Autodesk Inventor part; units mm, degrees
ref_plane "YZ Plane" through (0, 0, 0) normal (1, 0, 0) x (0, 1, 0)
ref_plane "XZ Plane" through (0, 0, 0) normal (0, 1, 0) x (-1, 0, 0)
ref_plane "XY Plane" through (0, 0, 0) normal (0, 0, 1) x (1, 0, 0)
sketch "main" plane through (0, 0, 0) normal (0, 0, 1) x (1, 0, 0)
  circle A0 centre (-11.2144, -104.2473) radius 2.1844
  circle A1 centre (1.4856, -104.2473) radius 2.1844
  circle A2 centre (48.9096, 6.9894) radius 2.1844
  circle A3 centre (-26.5889, 92.8058) radius 2.1844
  arc A4 (1.4856, -110.5973) -> (7.2979, -106.8047) centre (1.4856, -104.2473) ccw
  arc A5 (-17.0266, -101.6899) -> (-11.2144, -110.5973) centre (-11.2144, -104.2473) ccw
  line L0 (54.6905, 10.0319) -> (-22.1306, 97.3516)
  line L1 (55.7352, 3.2802) -> (7.2979, -106.8047)
  line L2 (-31.0925, 97.9248) -> (-34.2947, 95.1076)
  line L3 (-33.7837, 110.5973) -> (6.8178, 64.4472)
  line L4 (-17.0266, -101.6899) -> (6.006, -49.3432)
  line L5 (-34.8679, 86.1457) -> (-10.7088, 58.6849)
  arc A6 (-34.2947, 95.1076) -> (-34.8679, 86.1457) centre (-30.1004, 90.34) ccw
  arc A7 (-22.1306, 97.3516) -> (-31.0925, 97.9248) centre (-26.8981, 93.1573) ccw
  arc A8 (55.7352, 3.2802) -> (54.6905, 10.0319) centre (49.923, 5.8376) ccw
  arc A9 (6.006, -49.3432) -> (-10.7088, 58.6849) centre (-86.9901, -8.425) ccw
  line L6 (-11.2144, -110.5973) -> (1.4856, -110.5973)
  point P0 (16.4228, 13.0791)
  point P1 (-26.3249, 102.1192)
  point P2 (49.8339, -10.1318)
  dimension "d9" = 6.35
  dimension "d10" = 6.35
  dimension "d11" = 101.6
sketch "Sketch1" plane through (0, 0, 0) normal (1, 0, 0) x (0, 1, 0)
  circle A0 centre (78.4143, -41.889) radius 2.1
  circle A1 centre (0, 0) radius 2.1844
  circle A2 centre (0, -12.7) radius 2.1844
  circle A3 centre (111.2367, -60.124) radius 2.1844
  circle A4 centre (197.0531, 15.3746) radius 2.1844
  arc A5 (-6.35, -12.7) -> (-2.5574, -18.5123) centre (0, -12.7) ccw
  arc A6 (2.5574, 5.8123) -> (-6.35, 0) centre (0, 0) ccw
  line L0 (114.2793, -65.9049) -> (201.599, 10.9162)
  line L1 (107.5275, -66.9496) -> (-2.5574, -18.5123)
  line L2 (202.1722, 19.8781) -> (199.3549, 23.0804)
  line L3 (214.8446, 22.5693) -> (168.6945, -18.0321)
  line L4 (2.5574, 5.8123) -> (54.9042, -17.2203)
  line L5 (190.393, 23.6536) -> (162.9322, -0.5055)
  arc A7 (199.3549, 23.0804) -> (190.393, 23.6536) centre (194.5874, 18.886) ccw
  arc A8 (201.599, 10.9162) -> (202.1722, 19.8781) centre (197.4046, 15.6838) ccw
  arc A9 (107.5275, -66.9496) -> (114.2793, -65.9049) centre (110.0849, -61.1373) ccw
  arc A10 (54.9042, -17.2203) -> (162.9322, -0.5055) centre (95.8224, 75.7757) ccw
  line L6 (-6.35, 0) -> (-6.35, -12.7)
  point P0 (0, 0)
extrude "Extrusion1" add sketch "Sketch1" along normal blind 1.5875
properties part number "Support Gusset" material "Acetal Resin, White"
Check sheet for the modelled part. Datum: model origin and axes. Units: mm. A direction names the side the tool comes from. Round coordinates to 2 decimals unless told otherwise and drop trailing zeros. Loops run counter-clockwise (first coordinate to the right, second up) from the corner with the lowest first, then second, coordinate; pieces in that order, holes last. Notation, with made-up numbers: (-4.5, -24.75) -> (18.5, -24.75) arc R30 ccw to (18.5, 12.25) -> close; hole circle Ø9 at (15.5, 39). An arc over 180 degrees is marked (long way). Put each result on its own line as item: value. Start each with the question number.
1. Section check B-B (y = 0). Enter the section's corners in (x, z), plus the area to 3 significant figures.
2. Scan lines: probe 1 along Z at (x, y) = (1, 0); probe 2 along Y at (x, z) = (1, 0.5); probe 3 along Y at (x, z) = (1, 4.5). Record each from-to range of solid material in increasing order.
3. Section check C-C (x = 0.4). Enter the section's corners in (y, z), plus the area to 3 significant figures.
4. Access from +Z, -Z, +X, -X, +Y, -Y to the whole of each face (thin tool, end or side, straight path). Record for faces 4 (the face through (0.783, 2.084, -0.656)), 5 (the face through (0.78, 176.85, 11.74)).
5. Draft check along Y on faces 1 (the face through (0.78, 53.26, -43.07)), 2 (the face through (0.8, -3.5, 5.3)), 3 (the face through (0, 90, -28)). Enter one of: +Y half, -Y half, draft (parallel to the pull), parting line (faces both ways), or undercut.
6. Section check A-A (z = -20.5). Enter the section's corners in (x, y).
7. Section check D-D (z = -8.5). Enter the section's corners in (x, y), plus the area to 3 significant figures.
Findings:
1. outline: (0, -19.64) -> (1.59, -19.64) -> (1.59, -14.88) -> (0, -14.88) -> close; (0, -10.52) -> (1.59, -10.52) -> (1.59, -2.18) -> (0, -2.18) -> close; (0, 2.18) -> (1.59, 2.18) -> (1.59, 6.35) -> (0, 6.35) -> close
1. area: 27.4 mm^2
2. probe 1: z = -19.64 to -14.88, -10.52 to -2.18, 2.18 to 6.35
2. probe 2: y = -6.33 to -2.13, 2.13 to 14.63, 164.08 to 189.76
2. probe 3: y = -4.48 to 5.54, 168.62 to 194.31
3. outline: (-6.35, -12.7) arc R6.35 ccw to (-2.56, -18.51) -> (107.53, -66.95) arc R6.35 ccw to (114.28, -65.9) -> (201.6, 10.92) arc R6.35 ccw to (202.17, 19.88) -> (199.35, 23.08) arc R6.35 ccw to (190.39, 23.65) -> (162.93, -0.51) arc R101.6 cw to (54.9, -17.22) -> (2.56, 5.81) arc R6.35 ccw to (-6.35, 0) -> close; hole circle Ø4.37 at (0, -12.7); hole circle Ø4.37 at (0, 0); hole circle Ø4.2 at (78.41, -41.89); hole circle Ø4.37 at (111.24, -60.12); hole circle Ø4.37 at (197.05, 15.37)
3. area: 5,760 mm^2
4. face 4: +X, -X
4. face 5: +Z, +X, -X
5. face 1: -Y half
5. face 2: undercut
5. face 3: draft
6. outline: (0, 1.96) -> (1.59, 1.96) -> (1.59, 63.36) -> (0, 63.36) -> close; (0, 128.28) -> (1.59, 128.28) -> (1.59, 165.89) -> (0, 165.89) -> close
7. outline: (0, -6.35) -> (1.59, -6.35) -> (1.59, 35.09) -> (0, 35.09) -> close; (0, 152.57) -> (1.59, 152.57) -> (1.59, 179.53) -> (0, 179.53) -> close
7. area: 109 mm^2
